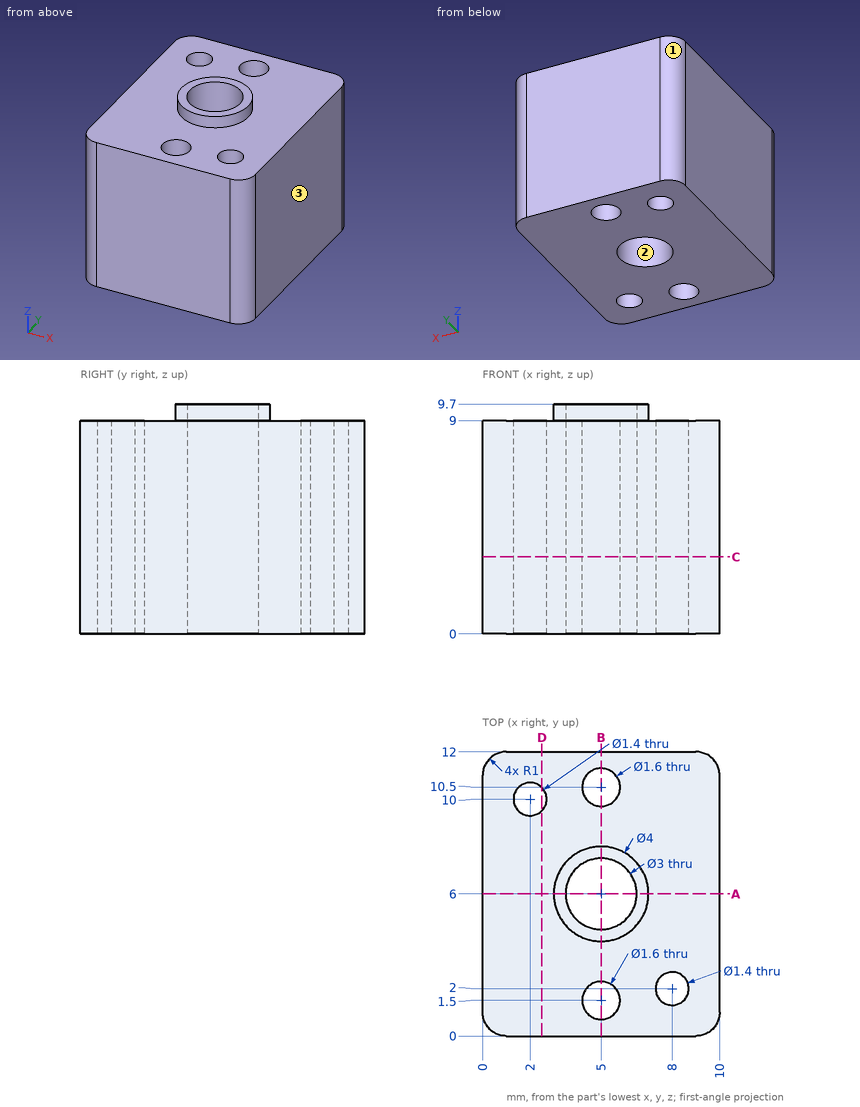
The figure shows three views and two pictorial views of one solid part (mm, origin at its lowest corner). Answer the questions. Coordinates: 2 decimals unless noted, no trailing zeros. Loops run counter-clockwise (first coordinate to the right, second up) from the corner with the lowest first, then second, coordinate; pieces in that order, holes last.
1) Find section D-D on x = 2.5. Write down the section's boundary in (y, z), then the cut area to 3 significant figures.
2) Find section B-B on x = 5. Write down the section's boundary in (y, z), then the cut area to 3 significant figures.
3) Find the intervals of material crossed by L1, parallel to Y at x = 5, z = 4; L2, parallel to Y at x = 8, z = 4; L3, parallel to X at y = 1.5, z = 3.75, in increasing order.
4) A flat-ended cylindrical pin translates along its axis: pin 1 Ø2 at (x, y) = (5, 10.5) entering from +Z. Find the tip coordinate at first contact, or state that the pin passes through.
5) Determine the mould class of the marked faces 1, 2 and 3 for opening direction Y: pulls with the +Y half, pulls with the -Y half, needs draft (parallel to the pull), parting line crosses it, or undercut.
6) Find section C-C on z = 3.25. Write down the section's boundary in (x, y), then the cut area to 3 significant figures.
7) Find section A-A on y = 6. Write down the section's boundary in (x, z).
Values:
1. outline: (0, 0) - (9.51, 0) - (9.51, 9) - (0, 9) - close; (10.49, 0) - (12, 0) - (12, 9) - (10.49, 9) - close
1. area: 99.2 mm2
2. outline: (0, 0) - (0.7, 0) - (0.7, 9) - (0, 9) - close; (2.3, 0) - (4.5, 0) - (4.5, 9.7) - (4, 9.7) - (4, 9) - (2.3, 9) - close; (7.5, 0) - (9.7, 0) - (9.7, 9) - (8, 9) - (8, 9.7) - (7.5, 9.7) - close; (11.3, 0) - (12, 0) - (12, 9) - (11.3, 9) - close
2. area: 52.9 mm2
3. L1: y = 0 to 0.7, 2.3 to 4.5, 7.5 to 9.7, 11.3 to 12
3. L2: y = 0 to 1.3, 2.7 to 12
3. L3: x = 0 to 4.2, 5.8 to 7.51, 8.49 to 10
4. pin 1: stops at z = 9
5. face 1: pulls with the +Y half
5. face 2: undercut
5. face 3: needs draft
6. outline: (0, 1) arc R1 ccw to (1, 0) - (9, 0) arc R1 ccw to (10, 1) - (10, 11) arc R1 ccw to (9, 12) - (1, 12) arc R1 ccw to (0, 11) - close; hole circle Ø1.4 at (2, 10); hole circle Ø3 at (5, 6); hole circle Ø1.6 at (5, 1.5); hole circle Ø1.6 at (5, 10.5); hole circle Ø1.4 at (8, 2)
6. area: 105 mm2
7. outline: (0, 0) - (3.5, 0) - (3.5, 9.7) - (3, 9.7) - (3, 9) - (0, 9) - close; (6.5, 0) - (10, 0) - (10, 9) - (7, 9) - (7, 9.7) - (6.5, 9.7) - close
